Source: three-view drawing plus pictorial views. Frame: mm from the lowest corner of the part. Give positions to 0.01 mm unless a question says otherwise; leave off trailing zeros. Loops run counter-clockwise (first coordinate to the right, second up) from the corner with the lowest first, then second, coordinate; pieces in that order, holes last. Notation, with made-up numbers: (83, 5.25) - (114, 5.25) arc R24 ccw to (114, 18.25) - close; hole circle Ø5 at (-26, 66.5). An arc over 180 degrees is marked (long way). Answer in a Markdown table with one row per item.
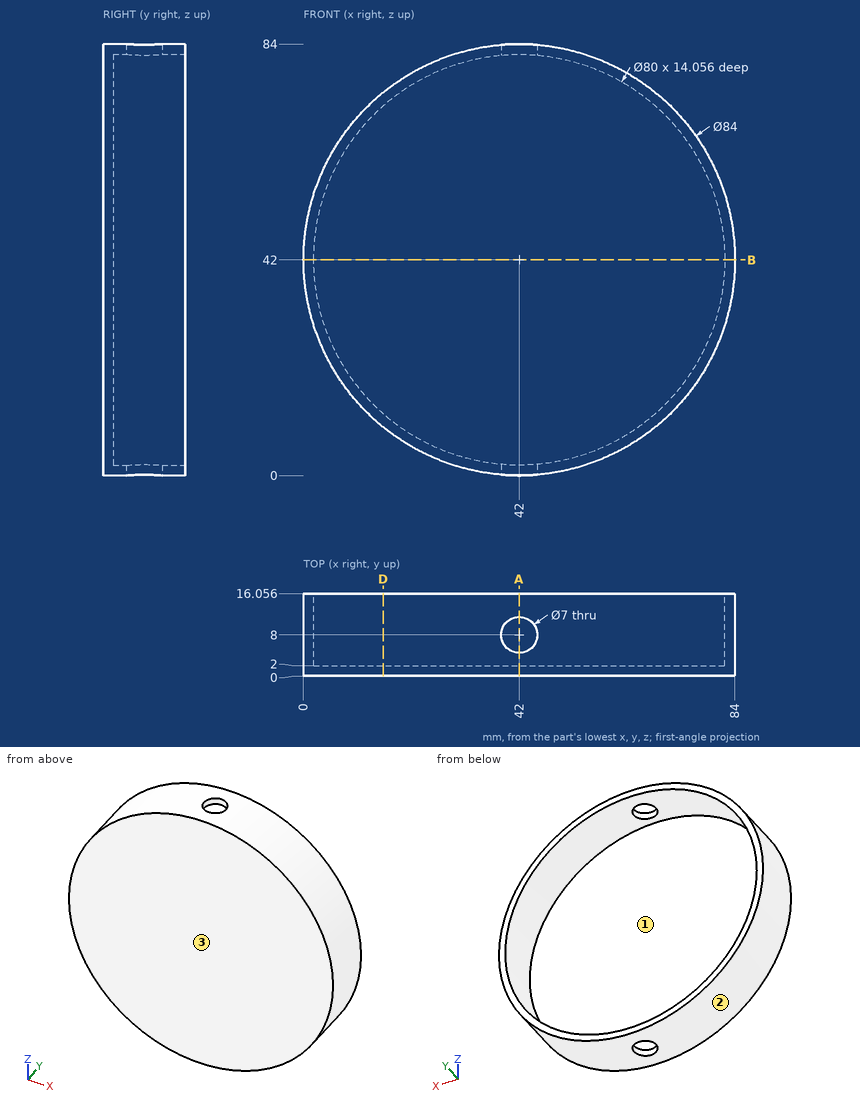
Q1. First-contact query: pin 1 (2 mm diameter, centred on y = 4.5, z = 51, fed in from +X); pin 2 (6 mm diameter, centred on x = 37, y = 13, fed in from +Z); pin 3 (6 mm diameter, centred on x = 38.5, y = 11.5, fed in from -Z). Flat tips, straight axial feed; report the tip coordinate or a pass-through.
Check values:
| item | result |
|---|---|
| pin 1 | x = 83.23 |
| pin 2 | z = 83.95 |
| pin 3 | z = 0 |
Q2. Material intervals for line 1 along Y through (x, z) = (27.5, 36); line 2 along X through (y, z) = (13.5, 77) (1 decimal); line 3 along Z through (x, y) = (23, 9.75), sorted ascending.
Check values:
| item | result |
|---|---|
| line 1 | 0 to 2 |
| line 2 | 18.8 to 22.6, 61.4 to 65.2 |
| line 3 | 4.54 to 6.8, 77.2 to 79.46 |
Q3. Cut plane B-B (z = 42). Output: boundary loops of the cut face in (x, y), and give its area (3 significant figures).
Check values:
| item | result |
|---|---|
| outline | (0, 0) - (84, 0) - (84, 16.06) - (82, 16.06) - (82, 2) - (2, 2) - (2, 16.06) - (0, 16.06) - close |
| area | 224 mm² |
Q4. Draft query along X for the marked faces 1, 2 and 3. Return one class per face: pulls with the +X half, pulls with the -X half, needs draft (parallel to the pull), parting line crosses it, or undercut.
Check values:
| item | result |
|---|---|
| face 1 | undercut |
| face 2 | parting line crosses it |
| face 3 | needs draft |
Q5. Cut plane D-D (x = 15.5). Output: boundary loops of the cut face in (y, z), and give its area (3 significant figures).
Check values:
| item | result |
|---|---|
| outline | (0, 9.42) - (16.06, 9.42) - (16.06, 12.04) - (2, 12.04) - (2, 71.96) - (16.06, 71.96) - (16.06, 74.58) - (0, 74.58) - close |
| area | 204 mm² |
Q6. Cut plane A-A (x = 42). Output: boundary loops of the cut face in (y, z).
Check values:
| item | result |
|---|---|
| outline | (0, 0) - (4.5, 0) - (4.5, 2) - (2, 2) - (2, 82) - (4.5, 82) - (4.5, 84) - (0, 84) - close; (11.5, 0) - (16.06, 0) - (16.06, 2) - (11.5, 2) - close; (11.5, 82) - (16.06, 82) - (16.06, 84) - (11.5, 84) - close |
